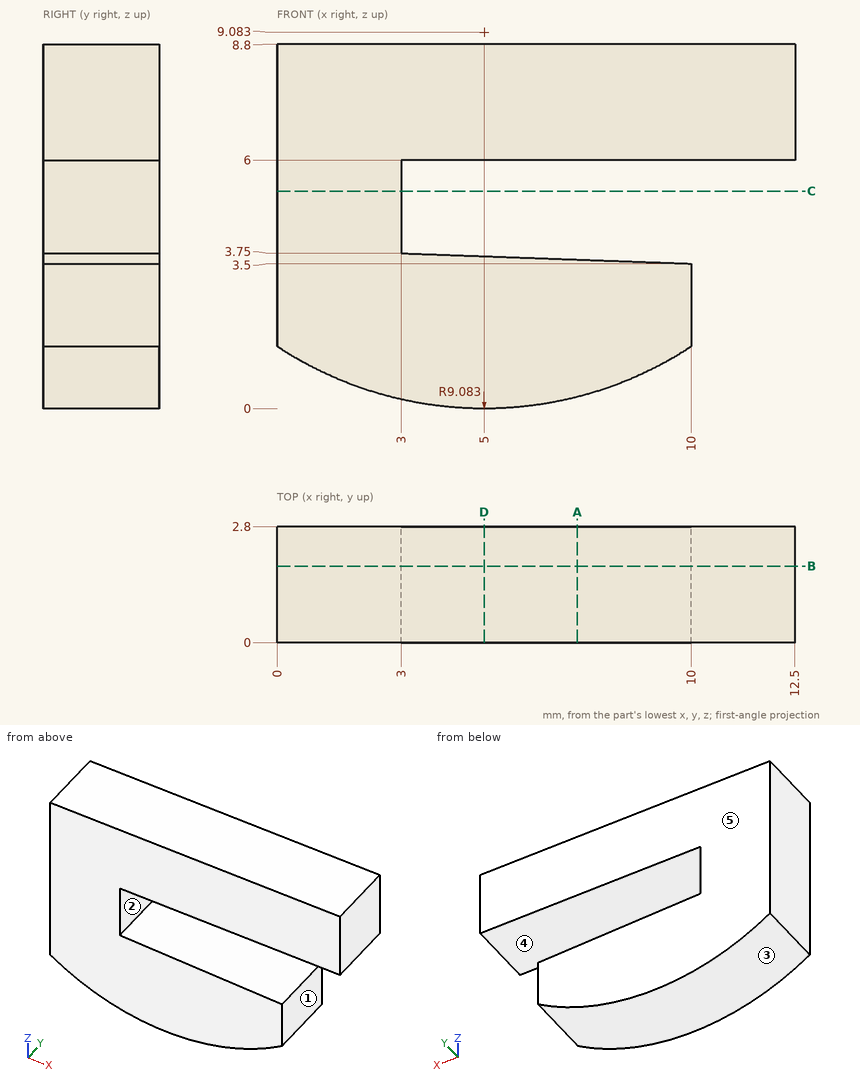
Input: dimensioned drawing with shaded views. Units: mm. Origin: part minimum x, y, z. A direction names the side the tool comes from. Coordinates: 2 decimals unless noted, no trailing zeros. Loops run counter-clockwise (first coordinate to the right, second up) from the corner with the lowest first, then second, coordinate; pieces in that order, holes last. Notation, with made-up numbers: M 66.5,-1.5 L 125.5,-1.5 A33 ccw 125.5,28.5 Z; hole C 46,26 d2. An arc over 180 degrees is marked long. One line per item, written item: value. Start each with the question number.
1) Cut plane D-D (x = 5). Return loops of the section in (y, z).
2) Pin query (flat end, axial travel): P1, Ø2, axis at x = 2, z = 5.5, coming from the -Y side; P2, Ø0.6, axis at y = 2, z = 2.5, coming from the +X side; P3, Ø0.8, axis at x = 9, y = 1.5, coming from the -Z side; P4, Ø0.7, axis at y = 1, z = 5, coming from the +X side. Return the tip coordinate at first contact, or that it passes through.
3) Cut plane B-B (y = 1.85). Return loops of the section in (x, z).
4) Cut plane A-A (x = 7.25). Return loops of the section in (y, z).
5) Cut plane C-C (z = 5.25). Return loops of the section in (x, y).
6) Reachability of the marked faces 4 and 5 from +Z, -Z, +X, -X, +Y, -Y: full face, straight path, thin tool, end or side. Return the list, or none.
7) Draft query along Z for the marked faces 1, 2 and 3. Return one class per face: released by +Z, released by -Z, zero draft, split by the parting line, or undercut.
8) Material intervals for L1, parallel to Z at x = 5.5, y = 2.05; L2, parallel to X at y = 1.9, z = 4; L3, parallel to Z at x = 10.5, y = 0.9, sorted ascending. Write a range as from..to.
Evaluation:
1. outline: M 0,0 L 2.8,0 L 2.8,3.68 L 0,3.68 Z; M 0,6 L 2.8,6 L 2.8,8.8 L 0,8.8 Z
2. P1: y = 0
2. P2: x = 10
2. P3: z = 0.74
2. P4: x = 3
3. outline: M 0,1.5 A9.08 ccw 10,1.5 L 10,3.5 L 3,3.75 L 3,6 L 12.5,6 L 12.5,8.8 L 0,8.8 Z
4. outline: M 0,0.28 L 2.8,0.28 L 2.8,3.6 L 0,3.6 Z; M 0,6 L 2.8,6 L 2.8,8.8 L 0,8.8 Z
5. outline: M 0,0 L 3,0 L 3,2.8 L 0,2.8 Z
6. face 4: +X, +Y, -Y
6. face 5: +Z, -Z, +X, -X, +Y
7. face 1: zero draft
7. face 2: undercut
7. face 3: released by -Z
8. L1: 0.01..3.66, 6..8.8
8. L2: 0..3
8. L3: 6..8.8
